Can you work these out from the model? Positions are in its coordinate system, mm. Give positions to 0.01 mm unless a question says otherwise; leave off trailing zeros. Loops run counter-clockwise (first coordinate to the right, second up) from the corner with the lowest first, then second, coordinate; pieces in that order, holes last. Notation, with made-up numbers: M 63,51.5 L 94,51.5 A6 ccw 94,58.5 Z; hole C 35,64 d5. An arc over 180 degrees is marked long. Answer as a JSON object with one key per item and string values.
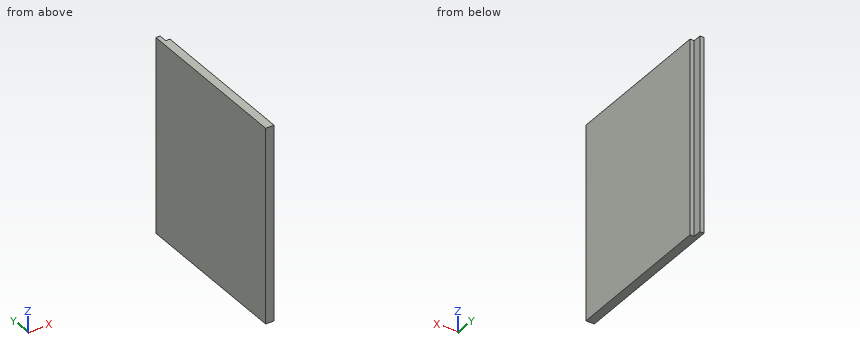
```python
from build123d import *

# Parameters (mm, degrees)
F0_W     = 234.95
F0_H     = 279.4
F2_DEPTH = 12.065
F3_W     = 12.065
F3_H     = 279.4
F4_DEPTH = 6.0325
F5_DEPTH = 0.4445


# Not quite as in the source:
# - a variable given as a bare number and used for a length is read in inches; the dataset says mm whatever the document's units were


with BuildPart() as f2:
    # F0 (on Right) → F2 (new body)
    with BuildSketch(Plane.YZ):
        Rectangle(F0_W, F0_H)
    extrude(amount=F2_DEPTH)

    # F3 (on face) → F4 (cut)
    with BuildSketch(Plane.YZ.offset(12.065)):
        with Locations((111.4425, 0)):
            Rectangle(F3_W, F3_H)
    extrude(amount=-F4_DEPTH, mode=Mode.SUBTRACT)

    # F5 (cut): a face of the model
    f5_faces = [f2.faces().sort_by_distance(p)[0] for p in [
        (5.9530149098, -2.9367649098, 139.7),
    ]]
    extrude(f5_faces, amount=-F5_DEPTH, mode=Mode.SUBTRACT)


solid = f2.part
```
1) Will these pins go through, and if not, where does the flat tip stop? pin 1 Ø5 at (x, z) = (9.5, 10.5) entering from +Y; pin 2 Ø3.5 at (y, z) = (111, 31) entering from +X.
Answer list:
{"pin 1": "y = 105.41", "pin 2": "x = 6.03"}
2) Please list where this line runs through material, in increasing order: line 1 along Y through (x, z) = (8, -13) (3 decimals). Write a range as from..to.
Answer list:
{"line 1": "-117.475..105.41"}
3) Suppose I cut it at A-A, the plane z = -2. Write out the boundary of the cut face in (x, y) (1 decimal).
Answer list:
{"outline": "M 0,-117.5 L 12.1,-117.5 L 12.1,105.4 L 6,105.4 L 6,117.5 L 0,117.5 Z"}
4) Suppose I cut it at B-B, the plane x = 10. Write out the boundary of the cut face in (y, z) (1 decimal), and give its area (3 significant figures).
Answer list:
{"outline": "M -117.5,-139.7 L 105.4,-139.7 L 105.4,139.3 L -117.5,139.3 Z", "area": "62,200 mm^2"}
